Can you work these out from the model? Positions are in its coordinate system, mm. Face numbers are marked on the shaded views. Give positions to 0.01 mm unless a question says otherwise; leave off trailing zeros. Loops run counter-clockwise (first coordinate to the right, second up) from the corner with the lowest first, then second, coordinate; pieces in that order, holes last. Notation, with made-up numbers: (-7.5, -15.5) -> (28.5, -15.5) arc R15 cw to (28.5, -7.5) -> close; hole circle Ø9 at (72, 53.5). An arc over 180 degrees is marked (long way). One line per question, with ' | ' between items.
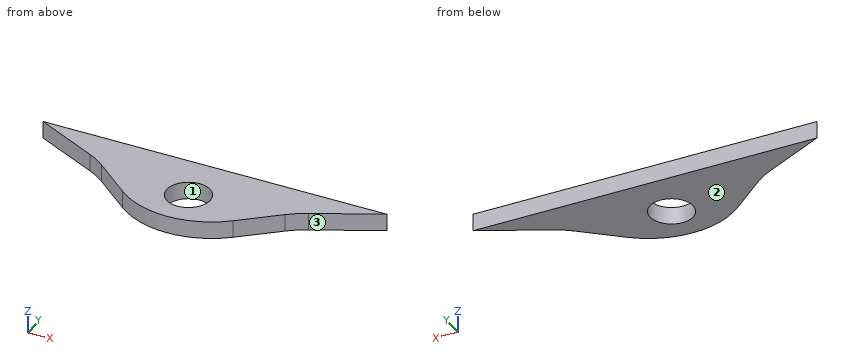
from build123d import *

# Parameters (mm, degrees)
SKETCH_1_R      = 2.5
EXTRUDE_1_DEPTH = 2
FILLET_1_R      = 10


with BuildPart() as part:
    # ｽｹｯﾁ1 → ﾎﾞｽ - 押し出し1 (new body)
    with BuildSketch(Plane.XY):
        Polygon((0, -7.832443736), (11.605504985, 1.905731217), (20, 6), (-20, 6), (-11.605504985, 1.905731217), align=None)
        Circle(SKETCH_1_R, mode=Mode.SUBTRACT)
    extrude(amount=EXTRUDE_1_DEPTH)

    # ﾌｨﾚｯﾄ1
    fillet_1_edges = [part.edges().sort_by_distance(p)[0] for p in [
        (-11.605504985, 1.905731217, 1),
        (11.605504985, 1.905731217, 1),
        (0, -7.832443736, 1),
    ]]
    fillet(fillet_1_edges, radius=FILLET_1_R)


solid = part.part
Q1. If we section it at A-A (x = 0): Write out the boundary of the cut face in (y, z).
Entries:
outline: (-4.78, 0) -> (-2.5, 0) -> (-2.5, 2) -> (-4.78, 2) -> close; (2.5, 0) -> (6, 0) -> (6, 2) -> (2.5, 2) -> close
Q2. If we section it at B-B (z = 1): Write out the boundary of the cut face in (x, y).
Entries:
outline: (-20, 6) -> (-12.71, 2.44) arc R10 cw to (-10.66, 1.12) -> (-6.43, -2.44) arc R10 ccw to (6.43, -2.44) -> (10.66, 1.12) arc R10 cw to (12.71, 2.44) -> (20, 6) -> close; hole circle Ø5 at (0, 0)
Q3. If we section it at D-D (x = -4.5): Write out the boundary of the cut face in (y, z), plus the area to 3 significant figures.
Entries:
outline: (-3.71, 0) -> (6, 0) -> (6, 2) -> (-3.71, 2) -> close | area: 19.4 mm²
Q4. For pin 1 Ø6 at (x, y) = (0, 0) entering from +Z, with a flat end and sliding along its axis, tell me the tip position at first contact or that it passes through.
Entries:
pin 1: z = 2
Q5. If we section it at C-C (y = -1.25): Write out the boundary of the cut face in (x, z).
Entries:
outline: (-7.84, 0) -> (-2.17, 0) -> (-2.17, 2) -> (-7.84, 2) -> close; (2.17, 0) -> (7.84, 0) -> (7.84, 2) -> (2.17, 2) -> close
Q6. If we mould it in two halves opening along X, with no side actions, what happens to the marked faces 1, 2 and 3? For each: pulls with the +X half, pulls with the -X half, needs draft (parallel to the pull), parting line crosses it, or undercut.
Entries:
face 1: undercut | face 2: needs draft | face 3: pulls with the +X half
Q7. If I drill on probe 1 along Y at (x, z) = (0, 1); probe 2 along X at (y, z) = (1.5, 0.85); probe 3 along X at (y, z) = (-0.5, 1.2), over which ranges is the centre line in solid material (lowest first)? Write a range as from..to.
Entries:
probe 1: -4.78..-2.5, 2.5..6 | probe 2: -11.15..-2, 2..11.15 | probe 3: -8.74..-2.45, 2.45..8.74
